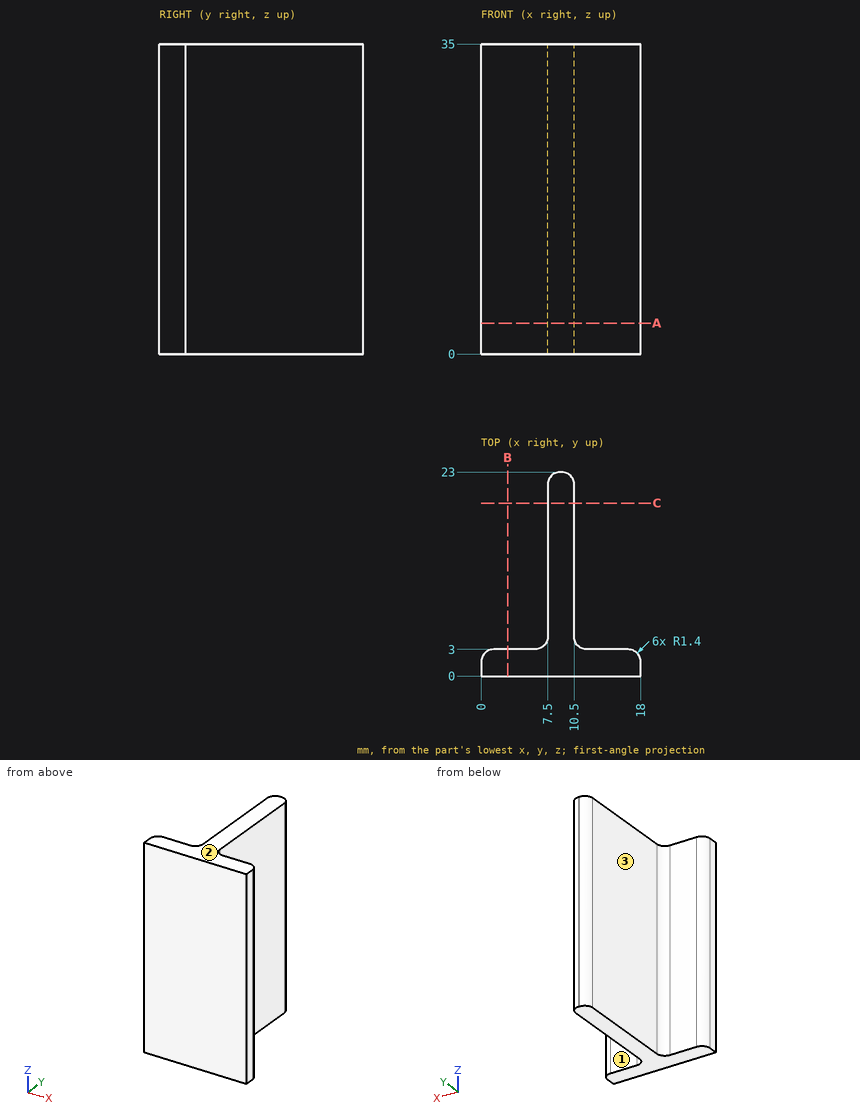
Job drawing, mm, ordinate dimensions from the low corner. One solid piece. A direction names the side the tool comes from. Coordinates: 2 decimals unless noted, no trailing zeros. Loops run counter-clockwise (first coordinate to the right, second up) from the corner with the lowest first, then second, coordinate; pieces in that order, holes last. Notation, with made-up numbers: (31.5, 23) - (64.5, 23) arc R13 cw to (64.5, 36) - close; hole circle Ø3 at (-11.5, 46.5). An arc over 180 degrees is marked (long way). Answer as a JSON object with one key per item and string values. Group by question number.
(1) Cut at C-C (y = 19.5). Give the cut face in (x, z).
(2) Probe line 1 along Y through (x, z) = (14, 30.5); line 2 along Y through (x, z) = (9.25, 30.5); line 3 along X through (y, z) = (14.5, 27). List the from-to ranges inside material, lowest first.
(3) Cut at B-B (x = 3). Give the cut face in (y, z).
(4) Flat gauge pins, fed straight in: pin 1 (5 mm diameter, centred on y = 12, z = 10, fed in from -X); pin 2 (1.4 mm diameter, centred on x = 3.5, z = 15.5, fed in from +Y); pin 3 (5 mm diameter, centred on y = 12.5, z = 22.5, fed in from +X). Where does each tip first touch, or does it go through?
(5) Cut at A-A (z = 3.5). Give the cut face in (x, y), then the cut area to 3 significant figures.
(6) Tool access for the marked faces 1, 2 and 3: list every direction of +Z, -Z, +X, -X, +Y, -Y with a clear straight run to the whole face (end or side of a thin tool).
Geometry says:
{
 "1": {"outline": "(7.5, 0) - (10.5, 0) - (10.5, 35) - (7.5, 35) - close"},
 "2": {"line 1": "y = 0 to 3", "line 2": "y = 0 to 22.99", "line 3": "x = 7.5 to 10.5"},
 "3": {"outline": "(0, 0) - (3, 0) - (3, 35) - (0, 35) - close"},
 "4": {"pin 1": "stops at x = 7.5", "pin 2": "stops at y = 3", "pin 3": "stops at x = 10.5"},
 "5": {"outline": "(0, 0) - (18, 0) - (18, 1.6) arc R1.4 ccw to (16.6, 3) - (11.9, 3) arc R1.4 cw to (10.5, 4.4) - (10.5, 21.6) arc R1.4 ccw to (9.1, 23) - (8.9, 23) arc R1.4 ccw to (7.5, 21.6) - (7.5, 4.4) arc R1.4 cw to (6.1, 3) - (1.4, 3) arc R1.4 ccw to (0, 1.6) - close", "area": "113 mm^2"},
 "6": {"face 1": "+Z, -Z, +X, +Y", "face 2": "+Z, +X, -X, +Y, -Y", "face 3": "+Z, -Z, -X, +Y"}
}
